Could you check a few things on this model? Use its own coordinates, in mm. A direction names the side the tool comes from. Round coordinates to 2 decimals unless told otherwise and drop trailing zeros. Loops run counter-clockwise (first coordinate to the right, second up) from the corner with the lowest first, then second, coordinate; pieces in that order, holes last. Notation, with made-up numbers: (9.5, 31.5) -> (52.5, 31.5) arc R11 ccw to (52.5, 35.5) -> close; hole circle Ø3 at (-9.5, 4). An arc over 180 degrees is marked (long way). Write each question's results on one line, items separated by ' | '. Start each with the question number.
1) Which directions (+Z, -Z, +X, -X, +Y, -Y) give clear straight access to the entire face, cutting with the end or side of a thin tool? Please do faces 4 (the flat face through (-4, 0, 0)), 5 (the flat face through (-26.752, -8, 1)), 6 (the cylindrical face through (-27.06, -11.11, -2.31)).
2) If I drill on probe 1 along Z at (x, y) = (-30, -32); probe 2 along Z at (x, y) = (-1, -4); probe 3 along Y at (x, z) = (-18.5, 2.25), over which ranges is the centre line in solid material (lowest first)?
3) For P1, Ø4, axis at y = -15.5, z = -3, coming from the +X side; P2, Ø6, axis at x = -4, y = -0.5, coming from the -Z side; P3, Ø1, axis at y = -25.5, z = -4.5, coming from the -X side, each with a flat end and sliding along its axis, tell me the tip position at first contact or that it passes through.
4) Imagine slicing it at B-B, the plane x = -8. List the corners of the cut face in (y, z) for me.
5) Imagine slicing it at C-C, the plane z = -4. List the corners of the cut face in (x, y) for me, plus the area to 3 significant figures.
6) Imagine slicing it at A-A, the plane z = 1.75. List the corners of the cut face in (x, y) for me.
7) We'd pull the mould along Y, two halves only. Please class faces 1 (the flat face through (-36, -23, -7.104)), 2 (the flat face through (-36.82, -36.36, -4.57)), 3 (the flat face through (-33.458, -30.835, -4.569)): pulls with the +Y half, pulls with the -Y half, needs draft (parallel to the pull), parting line crosses it, or undercut.
from build123d import *

# Parameters (mm, degrees)
ESQUISSE3_R             = 7
BOSS_EXTRU_2_DEPTH      = 5
BOSS_EXTRU_3_DEPTH      = 45
ENL_V_START             = -73.880031702
ENL_V_MAT_EXTRU_3_DEPTH = 78.880031702
ESQUISSE4_4_W           = 16.307493561
ESQUISSE4_4_H           = 7.104058167
ENL_V_MAT_EXTRU_4_DEPTH = 59.591870128
ENL_V_MAT_EXTRU_6_DEPTH = 58.24377063
ENL_V_MAT_EXTRU_7_DEPTH = 59.494096558


with BuildPart() as part:
    # Esquisse3 → Boss.-Extru.2 (new body)
    with BuildSketch(Plane.XY):
        Circle(ESQUISSE3_R)
    extrude(amount=BOSS_EXTRU_2_DEPTH)

    # Esquisse3_3 → Boss.-Extru.3 (add)
    with BuildSketch(Plane.XY):
        with BuildLine():
            ThreePointArc((-6.556240583, 2.452694319), (-31.795381091, -9.503990443), (-43.059714875, -35.059641647))
            Line((-43.059714875, -35.059641647), (-29.67043681, -37.846531887))
            Line((-29.67043681, -37.846531887), (-28.42882324, -31.881349224))
            Line((-28.42882324, -31.881349224), (-37.880972605, -29.913946449))
            ThreePointArc((-37.880972605, -29.913946449), (-26.825365644, -10.900303142), (-6.699170831, -2.030051767))
            ThreePointArc((-6.699170831, -2.030051767), (-6.99644453, 0.22307834), (-6.556240583, 2.452694319))
        make_face()
    boss_extru_3 = extrude(amount=BOSS_EXTRU_3_DEPTH)

    # Esquisse4 → Enl_v. mat.-Extru.3 (cut)
    with BuildSketch(Plane(origin=(0, 0, 0), x_dir=(1, 0, 0), z_dir=(0, 1, 0)).offset(ENL_V_START)):
        Polygon((-6.556240583, -21.643777245), (-6.556240583, -5), (-21.736227675, -5), (-21.736227675, -12.104058167), (-43.059714875, -12.104058167), (-43.059714875, -45), (-43.059714875, -53.527020644), (-6.425184121, -53.527020644), align=None)
    enl_v_mat_extru_3 = extrude(amount=ENL_V_MAT_EXTRU_3_DEPTH, mode=Mode.SUBTRACT)

    # Esquisse4_4 → Enl_v. mat.-Extru.4 (cut, through all)
    with BuildSketch(Plane(origin=(0, 0, 0), x_dir=(1, 0, 0), z_dir=(0, 1, 0))):
        with Locations((-34.905968095, -3.552029084)):
            Rectangle(ESQUISSE4_4_W, ESQUISSE4_4_H)
    enl_v_mat_extru_4 = extrude(amount=-ENL_V_MAT_EXTRU_4_DEPTH, mode=Mode.SUBTRACT)

    # Esquisse5 → Enl_v. mat.-Extru.6 (cut, through all)
    with BuildSketch(Plane(origin=(-7.540837864, -36.229046112, 0), x_dir=(0.9790175257089632, -0.2037760642340011, 0), z_dir=(0.2037760642340011, 0.9790175257089632, 0))):
        with BuildLine():
            Line((-22.326681436, -7.104058167), (-21.33566032, -7.104058167))
            Line((-21.33566032, -7.104058167), (-21.33566032, -12.104058167))
            Line((-21.33566032, -12.104058167), (-22.326681436, -12.104058167))
            ThreePointArc((-22.326681436, -12.104058167), (-22.079342596, -9.604058167), (-22.326681436, -7.104058167))
        make_face()
    enl_v_mat_extru_6 = extrude(amount=-ENL_V_MAT_EXTRU_6_DEPTH, mode=Mode.SUBTRACT)

    # Sym_trie1: Boss.-Extru.3, Enl_v. mat.-Extru.3, Enl_v. mat.-Extru.4, Enl_v. mat.-Extru.6 across plane
    add(boss_extru_3.mirror(Plane.XY.offset(2.5)))
    add(enl_v_mat_extru_3.mirror(Plane.XY.offset(2.5)), mode=Mode.SUBTRACT)
    add(enl_v_mat_extru_4.mirror(Plane.XY.offset(2.5)), mode=Mode.SUBTRACT)
    add(enl_v_mat_extru_6.mirror(Plane.XY.offset(2.5)), mode=Mode.SUBTRACT)

    # Esquisse6 → Enl_v. mat.-Extru.7 (cut, through all)
    with BuildSketch(Plane(origin=(0, 0, 0), x_dir=(1, 0, 0), z_dir=(0, 1, 0))):
        Polygon((-21.736227675, -5), (-29.704410318, -5), (-43.059714875, -7.104058167), (-43.059714875, -12.104058167), (-21.736227675, -12.104058167), align=None)
    extrude(amount=-ENL_V_MAT_EXTRU_7_DEPTH, mode=Mode.SUBTRACT)


solid = part.part
Checked values:
1) face 4: -Z, +X, +Y, -Y | face 5: +Z, -X, +Y, -Y | face 6: +Z, -Z
2) probe 1: -7.1 to -2.1 | probe 2: 0 to 5 | probe 3: -5.35 to -0.47
3) P1: x = -29.45 | P2: z = 0 | P3: x = -41.47
4) outline: (-2.19, 0) -> (2.3, 0) -> (2.3, 5) -> (-2.19, 5) -> close
5) outline: (-43.06, -35.06) -> (-30.41, -37.69) -> (-29.17, -31.73) -> (-37.88, -29.91) arc R35.55 cw to (-21.74, -7.11) -> (-21.74, -1.99) arc R40 ccw to start | area: 222 mm^2
6) outline: (-26.75, -10.84) arc R35.55 cw to (-6.7, -2.03) arc R7 ccw (long way) to (-6.56, 2.45) arc R40 ccw to (-26.75, -5.12) -> close
7) face 1: needs draft | face 2: pulls with the -Y half | face 3: undercut
